```python
from build123d import *

# Parameters (mm, degrees)
F0_R     = 11.1125
F1_DEPTH = 44.45
F2_R     = 6.35
F3_DEPTH = 88.9
F4_R     = 1.5584639764
F4_R_2   = 1.5569858866
F5_DEPTH = 12.7
F6_DEPTH = 12.7


with BuildPart() as f1:
    # F0 (on Front) → F1 (new body, symmetric)
    with BuildSketch(Plane.XZ):
        Circle(F0_R)
    extrude(amount=F1_DEPTH, both=True)

    # F2 (on face) → F3 (cut)
    with BuildSketch(Plane.XZ.offset(44.45)):
        Circle(F2_R)
    extrude(amount=-F3_DEPTH, mode=Mode.SUBTRACT)

    # F4 (on Right) → F5 (cut, symmetric)
    with BuildSketch(Plane.YZ):
        with Locations((12.2036093806, 0)):
            Circle(F4_R)
        with Locations((-9.5729407563, 0)):
            Circle(F4_R_2)
    extrude(amount=F5_DEPTH, both=True, mode=Mode.SUBTRACT)

    # F4 (on Right) → F6 (cut, symmetric)
    with BuildSketch(Plane.YZ):
        with Locations((12.2036093806, 0)):
            Circle(F4_R)
        with Locations((-9.5729407563, 0)):
            Circle(F4_R_2)
    extrude(amount=F6_DEPTH, both=True, mode=Mode.SUBTRACT)


solid = f1.part
```
Work out the finished part from the listing and answer in its coordinate system (mm). Give positions to 0.01 mm unless a question says otherwise; leave off trailing zeros. Loops run counter-clockwise (first coordinate to the right, second up) from the corner with the lowest first, then second, coordinate; pieces in that order, holes last. Notation, with made-up numbers: (51, -12) -> (79, -12) arc R29 cw to (79, 10) -> close; hole circle Ø4 at (-30.75, 20). An arc over 180 degrees is marked (long way). Use CSV: the item, a comma, the result in double quotes.
1. The part is cut by section D-D (x = -4.5). Write down the section's boundary in (y, z).
Found:
outline,"(-44.45, -10.16) -> (44.45, -10.16) -> (44.45, -4.48) -> (-44.45, -4.48) -> close; (-44.45, 4.48) -> (44.45, 4.48) -> (44.45, 10.16) -> (-44.45, 10.16) -> close"
2. The part is cut by section B-B (x = 0). Write down the section's boundary in (y, z), then the cut area to 3 significant figures.
Found:
outline,"(-44.45, -11.11) -> (44.45, -11.11) -> (44.45, -6.35) -> (-44.45, -6.35) -> close; (-44.45, 6.35) -> (44.45, 6.35) -> (44.45, 11.11) -> (-44.45, 11.11) -> close"
area,"847 mm^2"
3. Flat-ended cylindrical pins translate along their axes: pin 1 Ø1.9 at (y, z) = (12.2, 0) entering from +X; pin 2 Ø12 at (y, z) = (-34, 6.5) entering from +X; pin 3 Ø2 at (y, z) = (16.5, -6) entering from -X; pin 4 Ø10 at (x, y) = (6.5, -11.5) entering from -Z. Find the tip coordinate at first contact, or state that the pin passes through.
Found:
pin 1,"through"
pin 2,"x = 11.1"
pin 3,"x = -9.92"
pin 4,"z = -11.01"
4. The part is cut by section A-A (z = 0). Write down the section's boundary in (x, y), then the cut area to 3 significant figures.
Found:
outline,"(-11.11, -44.45) -> (-6.35, -44.45) -> (-6.35, -11.13) -> (-11.11, -11.13) -> close; (-11.11, -8.02) -> (-6.35, -8.02) -> (-6.35, 10.65) -> (-11.11, 10.65) -> close; (-11.11, 13.76) -> (-6.35, 13.76) -> (-6.35, 44.45) -> (-11.11, 44.45) -> close; (6.35, -44.45) -> (11.11, -44.45) -> (11.11, -11.13) -> (6.35, -11.13) -> close; (6.35, -8.02) -> (11.11, -8.02) -> (11.11, 10.65) -> (6.35, 10.65) -> close; (6.35, 13.76) -> (11.11, 13.76) -> (11.11, 44.45) -> (6.35, 44.45) -> close"
area,"787 mm^2"
5. Straight lines are drawn through the part: line 1 (Y direction, x = 8.35, z = 0); line 2 (X direction, y = -6, z = 0). For each, find the intervals that lie inside material, in ascending order.
Found:
line 1,"-44.45 to -11.13, -8.02 to 10.65, 13.76 to 44.45"
line 2,"-11.11 to -6.35, 6.35 to 11.11"
6. The mould has two halves that part along Y. Classify faces 1 (the cylindrical face through (6.057, -0.622, 1.907)), 2 (the flat face through (5, 44.45, -5)), 3 (the cylindrical face through (8.7, -8.1, 0.5)), 4 (the flat face through (5, -44.45, -5)): +Y half, -Y half, draft (parallel to the pull), parting line (faces both ways), or undercut.
Found:
face 1,"draft"
face 2,"+Y half"
face 3,"undercut"
face 4,"-Y half"
